Could you check a few things on this model? Use its own coordinates, in mm. A direction names the side the tool comes from. Coordinates: 2 decimals unless noted, no trailing zeros. Loops run counter-clockwise (first coordinate to the right, second up) from the corner with the lowest first, then second, coordinate; pieces in that order, holes last.
from build123d import *

# Parameters (mm, degrees)
BOSS_EXTRUDE1_DEPTH = 76.2
SKETCH2_R           = 7.332348419
SKETCH2_R_2         = 6.35
CUT_EXTRUDE1_DEPTH  = 11.1125
BOSS_EXTRUDE2_START = 9.525
SKETCH3_R           = 6.35
BOSS_EXTRUDE2_DEPTH = 9.525
SKETCH4_R           = 7.332348419
SKETCH4_R_2         = 5.9436
CUT_EXTRUDE2_DEPTH  = 0.889


with BuildPart() as part:
    # Sketch1 → Boss-Extrude1 (new, symmetric)
    with BuildSketch(Plane.XY):
        Polygon((3.684589596, -6.339332208), (7.332317533, 0.021282089), (3.647727937, 6.360614297), (-3.684589596, 6.339332208), (-7.332317533, -0.021282089), (-3.647727937, -6.360614297), align=None)
    extrude(amount=BOSS_EXTRUDE1_DEPTH, both=True)

    # Sketch2 → Cut-Extrude1 (cut)
    with BuildSketch(Plane.XY.offset(76.2)):
        Circle(SKETCH2_R)
        Circle(SKETCH2_R_2, mode=Mode.SUBTRACT)
    extrude(amount=-CUT_EXTRUDE1_DEPTH, mode=Mode.SUBTRACT)

    # Sketch3 → Boss-Extrude2 (add)
    with BuildSketch(Plane.XY.offset(76.2).offset(BOSS_EXTRUDE2_START)):
        Circle(SKETCH3_R)
    extrude(amount=-BOSS_EXTRUDE2_DEPTH)

    # Sketch4 → Cut-Extrude2 (cut)
    with BuildSketch(Plane.XY.offset(74.6125)):
        Circle(SKETCH4_R)
        Circle(SKETCH4_R_2, mode=Mode.SUBTRACT)
    extrude(amount=-CUT_EXTRUDE2_DEPTH, mode=Mode.SUBTRACT)


solid = part.part
(1) Which directions (+Z, -Z, +X, -X, +Y, -Y) give clear straight access to the entire face, cutting with the end or side of a thin tool? Please do faces 5 (the face through (-3, 6, 65.088)), 6 (the face through (3, 6, 65.088)), 7 (the face through (3, -6, 65.088)).
Answers:
face 5: +Z, -X, +Y
face 6: +Z, +X, +Y
face 7: +Z, +X, -Y
(2) We'd pull the mould along Z, two halves only. Please class faces 1 (the face through (0, 0, -76.2)), 2 (the face through (5.669, 1.785, 74.174)), 3 (the face through (-1.38, -6.2, 69.47)), 4 (the face through (-3, -6, 65.088)): +Z half, -Z half, draft (parallel to the pull), parting line (faces both ways), or undercut.
Answers:
face 1: -Z half
face 2: undercut
face 3: draft
face 4: +Z half
(3) For pin 1 (2 mm diameter, centred on y = -2.5, z = 44.5, fed in from +X); pin 2 (8 mm diameter, centred on x = 3.5, z = 68.5, fed in from -Y); pin 3 (4 mm diameter, centred on y = 2, z = 35, fed in from -X), each with a flat end and sliding along its axis, tell me the tip position at first contact or that it passes through.
Answers:
pin 1: stops at x = 6.46
pin 2: stops at y = -6.35
pin 3: stops at x = -7.32
(4) I need wall thicknesses on probe 1 along Z at (x, y) = (-4.25, 4.25) (1 decimal); probe 2 along Y at (x, z) = (1.5, 32); probe 3 along Y at (x, z) = (-3.25, -43.5). Which ranges of each line are inside material? Lowest first, please.
Answers:
probe 1: z = -76.2 to 73.7, 74.6 to 85.7
probe 2: y = -6.35 to 6.35
probe 3: y = -6.36 to 6.34
(5) Imagine slicing it at A-A, the plane z = -43. Write out the boundary of the cut face in (x, y).
Answers:
outline: (-7.33, -0.02) - (-3.65, -6.36) - (3.68, -6.34) - (7.33, 0.02) - (3.65, 6.36) - (-3.68, 6.34) - close
